from build123d import *

# Parameters (mm, degrees)
F1_DEPTH      = 170
F1_DEPTH_BACK = 30
F2_R          = 25
F3_DEPTH      = 60
F3_DEPTH_BACK = 60
F5_DEPTH      = 120.001
F5_DEPTH_BACK = 120.001
F6_R          = 20
F7_DEPTH      = 120.001
F7_DEPTH_BACK = 120.001
F8_SIZE       = 10


# Not quite as in the source:
# - a feature names something its author has since deleted; it is built from what else it names


with BuildPart() as f1:
    # F0 (on Right) → F1 (new body, two sides)
    with BuildSketch(Plane.YZ) as f1_sk:
        Polygon((-120, 95), (-120, -30), (-60, -30), (-60, 75), (0, 75), (60, 75), (60, -30), (120, -30), (120, 95), (0, 95), align=None)
    extrude(amount=F1_DEPTH)
    extrude(f1_sk.sketch, amount=-F1_DEPTH_BACK)

    # F2 (on Front) → F3 (join, two sides)
    with BuildSketch(Plane.XZ) as f3_sk:
        Circle(F2_R)
    extrude(amount=F3_DEPTH)
    extrude(f3_sk.sketch, amount=-F3_DEPTH_BACK)

    # F4 (on Front) → F5 (cut, two sides)
    with BuildSketch(Plane.XZ) as f5_sk:
        Polygon((170, -30), (170, 0), (135, 0), (100, 35), (90, 35), (25, -30), align=None)
    extrude(amount=-F5_DEPTH, mode=Mode.SUBTRACT)
    extrude(f5_sk.sketch, amount=F5_DEPTH_BACK, mode=Mode.SUBTRACT)

    # F6 (on Front) → F7 (cut, two sides)
    with BuildSketch(Plane.XZ) as f7_sk:
        with Locations((140, 35)):
            Circle(F6_R)
    extrude(amount=-F7_DEPTH, mode=Mode.SUBTRACT)
    extrude(f7_sk.sketch, amount=F7_DEPTH_BACK, mode=Mode.SUBTRACT)

    # F8
    f8_edges = [f1.edges().sort_by_distance(p)[0] for p in [
        (152.5, -60, 0),
        (152.5, 60, 0),
    ]]
    chamfer(f8_edges, length=F8_SIZE)


solid = f1.part
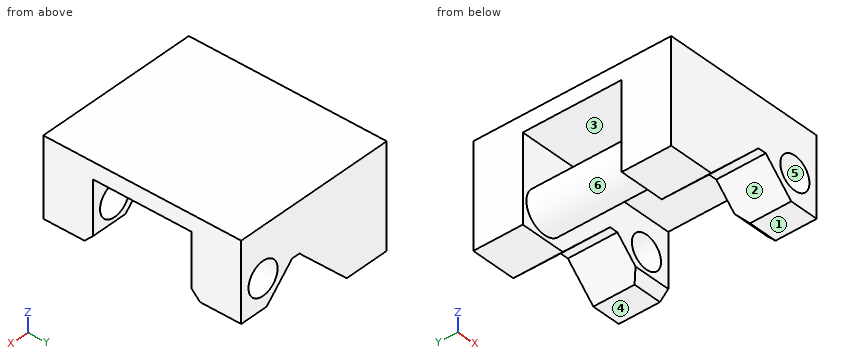
Verification items for the finished model (mm, model axes). Face numbers are marked on the shaded views. A direction names the side the tool comes from. Round coordinates to 2 decimals unless told otherwise and drop trailing zeros. Write each loop counter-clockwise with the first axis right and the second up, starting at its lowest first coordinate (ties: lowest second). Pieces come first, ordered by that corner, then holes.
(1) Section check C-C (y = -98). Enter the section's corners in (x, z).
Returned:
outline: (-30, -30) - (25, -30) - (90, 35) - (100, 35) - (135, 0) - (170, 0) - (170, 95) - (-30, 95) - close; hole circle Ø40 at (140, 35)
(2) Access from +Z, -Z, +X, -X, +Y, -Y to the whole of each face (thin tool, end or side, straight path). Record for the marked faces 1, 2 and 3.
Returned:
face 1: -Z, +X, +Y, -Y
face 2: -Z, +Y, -Y
face 3: +X, -X
(3) Section check A-A (z = 70.5). Enter the section's corners in (x, y).
Returned:
outline: (-30, -120) - (170, -120) - (170, -60) - (-30, -60) - close; (-30, 60) - (170, 60) - (170, 120) - (-30, 120) - close
(4) Section check D-D (x = 0). Enter the section's corners in (y, z).
Returned:
outline: (-120, -30) - (-60, -30) - (-60, -25) - (60, -25) - (60, -30) - (120, -30) - (120, 95) - (-120, 95) - close; hole (-60, 25) - (60, 25) - (60, 75) - (-60, 75) - close
(5) Section check B-B (x = 140). Enter the section's corners in (y, z), plus the area to 3 significant figures.
Returned:
outline: (-120, 0) - (-70, 0) - (-60, 10) - (-60, 15) - (-120, 15) - close; (-120, 55) - (-60, 55) - (-60, 75) - (60, 75) - (60, 55) - (120, 55) - (120, 95) - (-120, 95) - close; (60, 10) - (70, 0) - (120, 0) - (120, 15) - (60, 15) - close
area: 8,900 mm2
(6) Depth check by flat-ended pin: pin 1 Ø17.5 at (x, y) = (153, 91.5) entering from -Z; pin 2 Ø5 at (x, y) = (97, -95) entering from -Z; pin 3 Ø6 at (y, z) = (-21.5, -10) entering from +X. Enter the tip coordinate at first touch or a pass-through.
Returned:
pin 1: stops at z = 0
pin 2: stops at z = 35
pin 3: stops at x = 24
(7) Material ranges on line 1 (Y direction, x = -18, z = 47); line 2 (Z direction, x = 140, y = -106.5); line 3 (X direction, y = 75.5, z = 26), recorded low to high.
Returned:
line 1: y = -120 to -60, 60 to 120
line 2: z = 0 to 15, 55 to 95
line 3: x = -30 to 81, 109 to 122.14, 157.86 to 170
(8) Mould release check, pull along X, two halves, no side actions. Record for the marked faces 4, 5 and 6: pulls with the +X half, pulls with the -X half, needs draft (parallel to the pull), parting line crosses it, or undercut.
Returned:
face 4: needs draft
face 5: undercut
face 6: parting line crosses it
